from build123d import *

# Parameters (mm, degrees)
F1_DEPTH = 5


with BuildPart() as f1:
    # F0 (on Front) → F1 (new body)
    with BuildSketch(Plane.XZ):
        Polygon((-179.034567, 264.374884), (-173.507781, 264.35558), (-186.03374, 264.537622), align=None)
        Polygon((-179.034567, 264.374884), (-186.03374, 264.537622), (-187.878187, -263.855378), (7.564755, -264.537596), (98.705213, 154.081378), (118.589349, 154.011986), (161.871482, 153.860881), (187.878187, 255.596949), align=None)
        Polygon((-131.338066, -8.954973), (-159.987894, -8.854973), (-159.975677, -5.35498), (-131.325849, -5.45498), align=None, mode=Mode.SUBTRACT)
        Polygon((-148.081213, 11.980342), (-147.984185, 12.727559), (-147.794243, 13.456717), (-147.514412, 14.156309), (-147.149134, 14.815337), (-146.704101, 15.423363), (-146.186398, 15.970834), (-145.604154, 16.449091), (-144.966563, 16.850589), (-144.283659, 17.169028), (-143.566261, 17.399381), (-142.825622, 17.537989), (-142.073478, 17.582667), (-141.321638, 17.532731), (-140.58199, 17.388967), (-139.866192, 17.153611), (-139.185548, 16.830421), (-138.550777, 16.424453), (-137.971886, 15.942158), (-137.458018, 15.391079), (-137.017252, 14.779955), (-136.656572, 14.118412), (-136.381642, 13.416864), (-136.196807, 12.686411), (-136.10496, 11.938533), (-136.107602, 11.185068), (-136.204655, 10.437851), (-136.394571, 9.708693), (-136.674403, 9.009101), (-137.039706, 8.350072), (-137.484714, 7.742047), (-138.002416, 7.194575), (-138.584661, 6.716319), (-139.222251, 6.314796), (-139.905156, 5.996356), (-140.622553, 5.766029), (-141.363192, 5.627421), (-142.115362, 5.582742), (-142.867177, 5.632679), (-143.606825, 5.776443), (-144.322622, 6.011774), (-145.003266, 6.334989), (-145.638037, 6.740931), (-146.216929, 7.223252), (-146.730822, 7.77433), (-147.171562, 8.385454), (-147.532268, 9.046997), (-147.807197, 9.74852), (-147.992033, 10.478999), (-148.083854, 11.226851), align=None, mode=Mode.SUBTRACT)
        Polygon((-131.20718, 28.544799), (-159.857008, 28.644799), (-159.844791, 32.144792), (-131.194962, 32.044767), align=None, mode=Mode.SUBTRACT)
        Polygon((-32.229146, 120.487084), (-33.26351, 120.520638), (-59.115122, 126.551944), (-60.096933, 126.879198), (-60.962007, 127.447269), (-61.652506, 128.218159), (-62.122279, 129.140331), (-62.339906, 130.152115), (-62.290808, 131.185869), (-61.978311, 132.172481), (-61.423296, 133.045987), (-60.662845, 133.747993), (-59.747861, 134.231558), (-58.739456, 134.464323), (-57.705066, 134.43077), (-31.853454, 128.399489), (-30.871643, 128.07221), (-30.006569, 127.504139), (-29.31607, 126.733249), (-28.846297, 125.811077), (-28.628696, 124.799293), (-28.677768, 123.765539), (-28.990265, 122.778926), (-29.545305, 121.90542), (-30.305731, 121.203415), (-31.22074, 120.719875), align=None, mode=Mode.SUBTRACT)
    extrude(amount=F1_DEPTH)


solid = f1.part
Can you work these out from the model? Positions are in its coordinate system, mm. Round coordinates to 2 decimals unless told otherwise and drop trailing zeros. Loops run counter-clockwise (first coordinate to the right, second up) from the corner with the lowest first, then second, coordinate; pieces in that order, holes last. Notation, with made-up numbers: (-2, 81.5) - (25, 81.5) arc R19 cw to (25, 97.5) - close; hole circle Ø9 at (53.5, -39). An arc over 180 degrees is marked (long way). Write item = value, one per line. Start each with the question number.
(1) If we section it at C-C (z = -148.5): Please give me the cut outline in (x, y), and give its area (3 significant figures).
(2) If we section it at D-D (x = 143.5): Please give me the cut outline in (y, z).
(3) For P1, Ø1.5, axis at y = -2.5, z = 3.5, coming from the -X side; P2, Ø1.5, axis at y = -1.5, z = -26.5, coming from the +X side; P3, Ø1, axis at y = -1.5, z = -40, coming from the +X side, each with a flat end and sliding along its axis, tell me the tip position at first contact or that it passes through.
(4) If we mould it in two halves opening along Y, with no side actions, what happens to faces 1 (the face through (-44, 0, 62)), 2 (the face through (174.693, -2.465, 204.017)), 3 (the face through (-44, -5, 62))? For each: released by +Y, released by -Y, zero draft, split by the parting line, or undercut.
(5) If we section it at B-B (y = -3.7): Give the number of separate pieces and of enclosed holes in the cut face, and give its area (3 significant figures).
(6) If I drill on probe 1 along X at (y, z) = (-2.8, -51.5); probe 2 along X at (y, z) = (-3.35, -152); probe 3 along Z at (x, y) = (-114, -4.7), over which ranges is the centre line in solid material (lowest first)? Write a range as [from, to].
(7) If we section it at A-A (x = -42.5): Please give me the cut outline in (y, z).
Ans:
q1.outline = (-187.48, -5) - (32.83, -5) - (32.83, 0) - (-187.48, 0) - close
q1.area = 1,100 mm²
q2.outline = (-5, 153.93) - (0, 153.93) - (0, 256.66) - (-5, 256.66) - close
q3.P1 = -186.95
q3.P2 = 59.55
q3.P3 = 56.56
q4.face_1 = released by +Y
q4.face_2 = zero draft
q4.face_3 = released by -Y
q5.separate_pieces = 1
q5.enclosed_holes = 4
q5.area = 138,000 mm²
q6.probe_1 = [-187.14, 53.95]
q6.probe_2 = [-187.49, 32.07]
q6.probe_3 = [-264.11, 262.82]
q7.outline = (-5, -264.36) - (0, -264.36) - (0, 122.68) - (-5, 122.68) - close; (-5, 130.88) - (0, 130.88) - (0, 261.11) - (-5, 261.11) - close
